Work out the finished part from the listing and answer in its coordinate system (mm). Face numbers are marked on the shaded views. A direction names the side the tool comes from. Give positions to 0.01 mm unless a question says otherwise; leave off trailing zeros. Loops run counter-clockwise (first coordinate to the right, second up) from the corner with the lowest first, then second, coordinate; pieces in that order, holes last. Notation, with made-up numbers: (-14, 65) - (35, 65) arc R20 ccw to (35, 94) - close; hole circle Ø11 at (71, 65.5). An arc over 180 degrees is marked (long way). One line per item, written item: value.
from build123d import *

# Parameters (mm, degrees)
SKETCH_1_R          = 5.75
EXTRUDE_1_DEPTH     = 10
SKETCH_2_W          = 1.797928006
SKETCH_2_H          = 1.699859207
CUT_EXTRUDE_1_DEPTH = 5
SKETCH_3_R          = 7.5
SKETCH_3_R_2        = 7.143263017
EXTRUDE_2_DEPTH     = 10
SKETCH_4_R          = 7.5
EXTRUDE_3_DEPTH     = 1
FILLET_2_R          = 0.1


with BuildPart() as part:
    # Sketch 1 → Extrude 1 (new body)
    with BuildSketch(Plane(origin=(0, 0, 0), x_dir=(1, 0, 0), z_dir=(0, 1, 0))):
        with Locations(Location((0, 0, 0), (0, 0, 270))):
            Circle(SKETCH_1_R)
    extrude(amount=EXTRUDE_1_DEPTH)

    # Sketch 2 → Cut-Extrude 1 (cut)
    with BuildSketch(Plane(origin=(0, 10, 0), x_dir=(1, 0, 0), z_dir=(0, 1, 0))):
        with BuildLine():
            Line((0.212482401, -2.577588151), (0.212482401, -1.299411605))
            Line((0.212482401, -1.299411605), (-0.212482401, -1.299411605))
            Line((-0.212482401, -1.299411605), (-0.212482401, -2.577588151))
            ThreePointArc((-0.212482401, -2.577588151), (-0.457654402, -2.982926011), (-0.212482401, -3.388263872))
            Line((-0.212482401, -3.388263872), (-0.212482401, -4.666440418))
            Line((-0.212482401, -4.666440418), (0.212482401, -4.666440418))
            Line((0.212482401, -4.666440418), (0.212482401, -3.388263872))
            ThreePointArc((0.212482401, -3.388263872), (0.457654402, -2.982926011), (0.212482401, -2.577588151))
        make_face()
        with Locations((0, 5.04237082)):
            Rectangle(SKETCH_2_W, SKETCH_2_H)
        with BuildLine():
            Line((-1.343166429, -2.210206641), (-0.591873105, -1.176140093))
            Line((-0.591873105, -1.176140093), (-0.935676851, -0.92635205))
            Line((-0.935676851, -0.92635205), (-1.686970175, -1.960418597))
            ThreePointArc((-1.686970175, -1.960418597), (-2.123570107, -2.144235328), (-2.163473408, -2.616269032))
            Line((-2.163473408, -2.616269032), (-2.914766732, -3.65033558))
            Line((-2.914766732, -3.65033558), (-2.570962985, -3.900123623))
            Line((-2.570962985, -3.900123623), (-1.819669661, -2.866057075))
            ThreePointArc((-1.819669661, -2.866057075), (-1.38306973, -2.682240344), (-1.343166429, -2.210206641))
        make_face()
        with BuildLine():
            Line((-2.385771335, -0.998601315), (-1.170153201, -0.603623041))
            Line((-1.170153201, -0.603623041), (-1.301474547, -0.199457497))
            Line((-1.301474547, -0.199457497), (-2.517092681, -0.594435771))
            ThreePointArc((-2.517092681, -0.594435771), (-2.978354209, -0.48651963), (-3.288091107, -0.844948346))
            Line((-3.288091107, -0.844948346), (-4.50370924, -1.23992662))
            Line((-4.50370924, -1.23992662), (-4.372387895, -1.644092164))
            Line((-4.372387895, -1.644092164), (-3.156769761, -1.24911389))
            ThreePointArc((-3.156769761, -1.24911389), (-2.695508233, -1.357030032), (-2.385771335, -0.998601315))
        make_face()
        with BuildLine():
            Line((2.517092681, -0.594435771), (1.301474547, -0.199457497))
            Line((1.301474547, -0.199457497), (1.170153201, -0.603623041))
            Line((1.170153201, -0.603623041), (2.385771335, -0.998601315))
            ThreePointArc((2.385771335, -0.998601315), (2.695508233, -1.357030032), (3.156769761, -1.24911389))
            Line((3.156769761, -1.24911389), (4.372387895, -1.644092164))
            Line((4.372387895, -1.644092164), (4.50370924, -1.23992662))
            Line((4.50370924, -1.23992662), (3.288091107, -0.844948346))
            ThreePointArc((3.288091107, -0.844948346), (2.978354209, -0.48651963), (2.517092681, -0.594435771))
        make_face()
        with BuildLine():
            Line((1.686970175, -1.960418597), (0.935676851, -0.92635205))
            Line((0.935676851, -0.92635205), (0.591873105, -1.176140093))
            Line((0.591873105, -1.176140093), (1.343166429, -2.210206641))
            ThreePointArc((1.343166429, -2.210206641), (1.38306973, -2.682240344), (1.819669661, -2.866057075))
            Line((1.819669661, -2.866057075), (2.570962985, -3.900123623))
            Line((2.570962985, -3.900123623), (2.914766732, -3.65033558))
            Line((2.914766732, -3.65033558), (2.163473408, -2.616269032))
            ThreePointArc((2.163473408, -2.616269032), (2.123570107, -2.144235328), (1.686970175, -1.960418597))
        make_face()
    extrude(amount=-CUT_EXTRUDE_1_DEPTH, mode=Mode.SUBTRACT)



with BuildPart() as body_2:
    # Sketch 3 → Extrude 2 (new body)
    with BuildSketch(Plane(origin=(0, 0, 0), x_dir=(1, 0, 0), z_dir=(0, 1, 0))):
        with Locations(Location((0, 0, 0), (0, 0, 270))):
            Circle(SKETCH_3_R)
        with Locations(Location((0, 0, 0), (0, 0, 270))):
            Circle(SKETCH_3_R_2, mode=Mode.SUBTRACT)
    extrude(amount=EXTRUDE_2_DEPTH)


with BuildPart() as part_1:
    add(part.part)

    add(body_2.part)  # Extrude 3 merges body 2
    # Sketch 4 → Extrude 3 (add)
    with BuildSketch(Plane.XZ):
        with Locations(Location((0, 0, 0), (0, 0, 90))):
            Circle(SKETCH_4_R)
    extrude(amount=EXTRUDE_3_DEPTH)

    # Fillet 2
    fillet_2_edges = [part_1.edges().sort_by_distance(p)[0] for p in [
        (0, 10, -7.5),
        (0, 10, -7.143263017),
    ]]
    fillet(fillet_2_edges, radius=FILLET_2_R)


solid = part_1.part
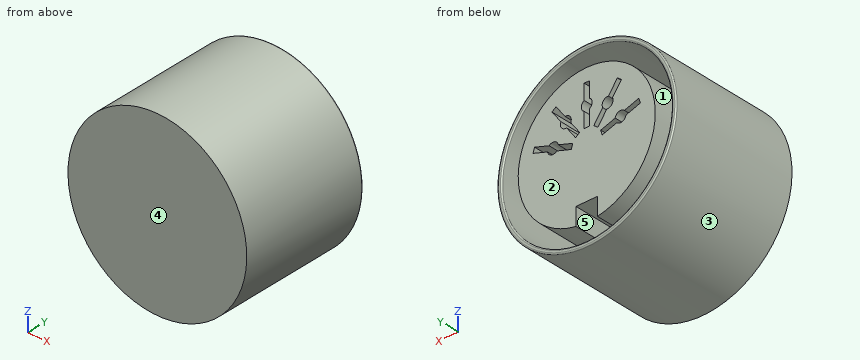
1. For the marked faces 1 and 2, determine the directions among +Z, -Z, +X, -X, +Y, -Y from which every point of the face is accessible in a straight line to the end or side of a thin tool.
Output:
face 1: +Y
face 2: +Z, -Z, +X, -X, +Y
2. Find the intervals of material crossed by line 1 along X through (y, z) = (3.25, 0); line 2 along Z through (x, y) = (-0.25, 8.5); line 3 along Z through (x, y) = (4.75, 9), in increasing order.
Output:
line 1: x = -7.5 to -7.14, -5.75 to 5.75, 7.14 to 7.5
line 2: z = -7.5 to -7.14, -4.19 to 2.6, 3.37 to 5.74, 7.14 to 7.5
line 3: z = -5.8 to -5.34, -3.24 to 3.24, 5.34 to 5.8
3. Section A-A (y = 3) is taken. Write down the section's boundary in (x, z), and give its area (3 significant figures).
Output:
outline: circle Ø15 at (0, 0); circle Ø11.5 at (0, 0); hole circle Ø14.29 at (0, 0)
area: 120 mm²
4. Section B-B (z = 0) is taken. Write down the section's boundary in (x, y), and give its area (3 significant figures).
Output:
outline: (-7.5, -1) - (7.5, -1) - (7.5, 9.9) arc R0.1 ccw to (7.4, 10) - (7.24, 10) arc R0.1 ccw to (7.14, 9.9) - (7.14, 0) - (5.75, 0) - (5.75, 10) - (-5.75, 10) - (-5.75, 0) - (-7.14, 0) - (-7.14, 9.9) arc R0.1 ccw to (-7.24, 10) - (-7.4, 10) arc R0.1 ccw to (-7.5, 9.9) - close
area: 137 mm²
5. Flat-ended cylindrical pins translate along their axes: pin 1 Ø1 at (y, z) = (4, -3) entering from +X; pin 2 Ø1.4 at (y, z) = (7, 4.5) entering from -X; pin 3 Ø1 at (y, z) = (5.5, 1.5) entering from -X. Find the tip coordinate at first contact, or state that the pin passes through.
Output:
pin 1: stops at x = 7.07
pin 2: stops at x = -6.47
pin 3: stops at x = -7.43
6. Section C-C (x = 0) is taken. Write down the section's boundary in (y, z).
Output:
outline: (-1, -7.5) - (9.9, -7.5) arc R0.1 ccw to (10, -7.4) - (10, -7.24) arc R0.1 ccw to (9.9, -7.14) - (0, -7.14) - (0, -5.75) - (5, -5.75) - (5, -4.19) - (10, -4.19) - (10, 1.3) - (5, 1.3) - (5, 4.67) - (10, 4.67) - (10, 5.75) - (0, 5.75) - (0, 7.14) - (9.9, 7.14) arc R0.1 ccw to (10, 7.24) - (10, 7.4) arc R0.1 ccw to (9.9, 7.5) - (-1, 7.5) - close
7. The mould has two halves that part along Z. Classify the marked faces 3, 4 and 5: released by +Z, released by -Z, zero draft, split by the parting line, or undercut.
Output:
face 3: split by the parting line
face 4: zero draft
face 5: undercut
